from build123d import *

# Parameters (mm, degrees)
SKETCH2_W           = 106.68
SKETCH2_H           = 38.1
BOSS_EXTRUDE1_DEPTH = 1.5748
SKETCH3_R           = 1.9
CUT_EXTRUDE1_DEPTH  = 2.5748
SKETCH4_W           = 82.55
SKETCH4_H           = 31.75
BOSS_EXTRUDE2_DEPTH = 22.2504
BOSS_EXTRUDE3_DEPTH = 1.5875
SKETCH7_R           = 0.9
SKETCH7_R_2         = 0.6
BOSS_EXTRUDE4_DEPTH = 3.175
BOSS_EXTRUDE5_DEPTH = 6.35


with BuildPart() as part:
    # Sketch2 → Boss-Extrude1 (new body)
    with BuildSketch(Plane(origin=(0, 0, 0), x_dir=(1, 0, 0), z_dir=(0, 1, 0))):
        Rectangle(SKETCH2_W, SKETCH2_H)
    extrude(amount=-BOSS_EXTRUDE1_DEPTH)

    # Sketch3 → Cut-Extrude1 (cut, through all)
    with BuildSketch(Plane(origin=(0, 0, 0), x_dir=(1, 0, 0), z_dir=(0, 1, 0))):
        with Locations((-48.635996958, 12.660327112)):
            Circle(SKETCH3_R)
        with Locations((-48.635996958, -12.731304513)):
            Circle(SKETCH3_R)
        with Locations((48.5775, 12.660327112)):
            Circle(SKETCH3_R)
        with Locations((48.5775, -12.731304513)):
            Circle(SKETCH3_R)
    extrude(amount=-CUT_EXTRUDE1_DEPTH, mode=Mode.SUBTRACT)

    # Sketch4 → Boss-Extrude2 (add)
    with BuildSketch(Plane(origin=(0, 0, 0), x_dir=(1, 0, 0), z_dir=(0, 1, 0))):
        Rectangle(SKETCH4_W, SKETCH4_H)
    extrude(amount=BOSS_EXTRUDE2_DEPTH)

    # Sketch5 → Boss-Extrude3 (add)
    with BuildSketch(Plane(origin=(41.275, 0, 0), x_dir=(0, 0, -1), z_dir=(1, 0, 0))):
        with BuildLine():
            Line((-12.543194793, 6.326748643), (12.543194793, 6.326748643))
            ThreePointArc((12.543194793, 6.326748643), (13.427078269, 6.692865167), (13.793194793, 7.576748643))
            Line((13.793194793, 7.576748643), (13.793194793, 18.610210685))
            ThreePointArc((13.793194793, 18.610210685), (13.427078269, 19.494094161), (12.543194793, 19.860210685))
            Line((12.543194793, 19.860210685), (-12.543194793, 19.860210685))
            ThreePointArc((-12.543194793, 19.860210685), (-13.427078269, 19.494094161), (-13.793194793, 18.610210685))
            Line((-13.793194793, 18.610210685), (-13.793194793, 7.576748643))
            ThreePointArc((-13.793194793, 7.576748643), (-13.427078269, 6.692865167), (-12.543194793, 6.326748643))
        make_face()
    extrude(amount=BOSS_EXTRUDE3_DEPTH)

    # Sketch7 → Boss-Extrude4 (add)
    with BuildSketch(Plane(origin=(42.8625, 0, 0), x_dir=(0, 0, -1), z_dir=(1, 0, 0))):
        with Locations((11.961268356, 13.093479664)):
            Circle(SKETCH7_R)
        with Locations((11.961268356, 13.093479664)):
            Circle(SKETCH7_R_2, mode=Mode.SUBTRACT)
        with Locations((-12.038731644, 13.093479664)):
            Circle(SKETCH7_R)
        with Locations((-12.038731644, 13.093479664)):
            Circle(SKETCH7_R_2, mode=Mode.SUBTRACT)
    extrude(amount=BOSS_EXTRUDE4_DEPTH)

    # Sketch8 → Boss-Extrude5 (add)
    with BuildSketch(Plane(origin=(42.8625, 0, 0), x_dir=(0, 0, -1), z_dir=(1, 0, 0))):
        with BuildLine():
            Line((-8.331799028, 16.906508091), (-5.797073634, 9.718080521))
            ThreePointArc((-5.797073634, 9.718080521), (-5.568701271, 9.415761232), (-5.207643796, 9.30092052))
            Line((-5.207643796, 9.30092052), (5.207643796, 9.30092052))
            ThreePointArc((5.207643796, 9.30092052), (5.568701271, 9.415761232), (5.797073634, 9.718080521))
            Line((5.797073634, 9.718080521), (8.331799028, 16.906508091))
            ThreePointArc((8.331799028, 16.906508091), (8.252528477, 17.475405565), (7.742369189, 17.73934809))
            Line((7.742369189, 17.73934809), (-7.742369189, 17.73934809))
            ThreePointArc((-7.742369189, 17.73934809), (-8.252528477, 17.475405565), (-8.331799028, 16.906508091))
        make_face()
    extrude(amount=BOSS_EXTRUDE5_DEPTH)


solid = part.part
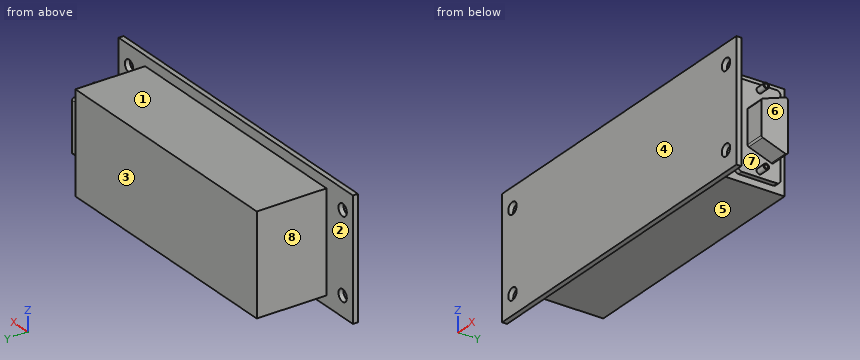
Check sheet for the modelled part. Datum: model origin and axes. Units: mm. Face numbers are marked on the shaded views. A direction names the side the tool comes from. Give positions to 0.01 mm unless a question says otherwise; leave off trailing zeros. Write each loop counter-clockwise with the first axis right and the second up, starting at its lowest first coordinate (ties: lowest second). Pieces come first, ordered by that corner, then holes. Notation, with made-up numbers: (81, 36.25) -> (92, 36.25) arc R15 cw to (92, 40.25) -> close; hole circle Ø5 at (-33.75, 35). An arc over 180 degrees is marked (long way). Use one line per item in the form item = value. Start each with the question number.
1. Section check D-D (y = 1.5). Record the cut outline in (x, z) (3 decimals), and give its area (3 significant figures).
2. Mould release check, pull along Y, two halves, no side actions. Record for the marked faces 1, 2, 3 and 4: pulls with the +Y half, pulls with the -Y half, needs draft (parallel to the pull), parting line crosses it, or undercut.
3. Go/stop test with flat-tipped pins: P1, Ø4, axis at x = 23.5, y = 15.5, coming from the -Z side (3 decimals); P2, Ø4, axis at y = 15, z = -12.5, coming from the -X side (3 decimals); P3, Ø5, axis at x = 48.58, z = -12.66, coming from the +Y side. Record where each tip stops, or that it passes through.
4. Thickness scan on line 1 along Z through (x, y) = (-25, 0.75) (3 decimals); line 2 along X through (y, z) = (6, 15) (3 decimals); line 3 along X through (y, z) = (8, 11) (1 decimal). Record the ranges inside material, lowest first. Write a range as from..to.
5. Section check C-C (y = 15). Record the cut outline in (x, z) (1 decimal), and give its area (3 significant figures).
6. Section check B-B (x = 3.5). Record the cut outline in (y, z) (3 decimals).
7. Section check A-A (z = -2). Record the cut outline in (x, y) (1 decimal).
8. Access from +Z, -Z, +X, -X, +Y, -Y to the whole of each face (thin tool, end or side, straight path). Record for the marked faces 5, 6, 7 and 8.
Conclusion:
q1.outline = (-41.275, -15.875) -> (41.275, -15.875) -> (41.275, 15.875) -> (-41.275, 15.875) -> close
q1.area = 2,620 mm²
q2.face_1 = needs draft
q2.face_2 = undercut
q2.face_3 = pulls with the +Y half
q2.face_4 = pulls with the -Y half
q3.P1 = -15.875
q3.P2 = -41.275
q3.P3 = 0
q4.line_1 = -15.875..15.875
q4.line_2 = -41.275..41.275
q4.line_3 = -41.3..42.9
q5.outline = (-41.3, -15.9) -> (41.3, -15.9) -> (41.3, -13.8) -> (42.9, -13.8) -> (42.9, -7.7) -> (49.2, -7.7) -> (49.2, 7.7) -> (42.9, 7.7) -> (42.9, 13.8) -> (41.3, 13.8) -> (41.3, 15.9) -> (-41.3, 15.9) -> close
q5.area = 2,760 mm²
q6.outline = (-1.575, -19.05) -> (0, -19.05) -> (0, -15.875) -> (22.25, -15.875) -> (22.25, 15.875) -> (0, 15.875) -> (0, 19.05) -> (-1.575, 19.05) -> close
q7.outline = (-53.3, -1.6) -> (53.3, -1.6) -> (53.3, 0) -> (41.3, 0) -> (41.3, 6.3) -> (42.9, 6.3) -> (42.9, 9.3) -> (49.2, 9.3) -> (49.2, 17.7) -> (42.9, 17.7) -> (42.9, 19.9) -> (41.3, 19.9) -> (41.3, 22.3) -> (-41.3, 22.3) -> (-41.3, 0) -> (-53.3, 0) -> close
q8.face_5 = -Z, +X, -X, +Y
q8.face_6 = +Z, -Z, +X, +Y
q8.face_7 = +X
q8.face_8 = +Z, -Z, -X, +Y
